from build123d import *

# Parameters (mm, degrees)
SKETCH_1_W          = 60
SKETCH_1_H          = 60
EXTRUDE_1_DEPTH     = 37
SKETCH_2_W          = 56
SKETCH_2_H          = 56
EXTRUDE_2_DEPTH     = 49
CUT_EXTRUDE_1_DEPTH = 49
SKETCH_4_R          = 2
CUT_EXTRUDE_2_DEPTH = 49
FILLET_1_R          = 2
SKETCH_5_R          = 27
CUT_EXTRUDE_3_DEPTH = 1
SKETCH_6_R          = 12
EXTRUDE_3_DEPTH     = 4
SKETCH_7_R          = 4
EXTRUDE_4_DEPTH     = 27
SKETCH_8_W          = 5.291502622
SKETCH_8_H          = 3.956308335
CUT_EXTRUDE_4_DEPTH = 27
FILLET_2_R          = 1
FILLET_3_R          = 3


with BuildPart() as part:
    # Эскиз1 → Бобышка-Вытянуть1 (new body)
    with BuildSketch(Plane.XY):
        with Locations((0.572032188, -6.927630122)):
            Rectangle(SKETCH_1_W, SKETCH_1_H)
    extrude(amount=EXTRUDE_1_DEPTH)

    # Эскиз2 → Бобышка-Вытянуть2 (add)
    with BuildSketch(Plane.XY.offset(37)):
        with Locations((0.572032188, -6.927630122)):
            Rectangle(SKETCH_2_W, SKETCH_2_H)
    extrude(amount=EXTRUDE_2_DEPTH)

    # Эскиз3 → Вырез-Вытянуть1 (cut)
    with BuildSketch(Plane.XY.offset(86)):
        with BuildLine():
            Line((-19.176705154, 17.82110722), (-19.176705154, 21.072369878))
            Line((-19.176705154, 21.072369878), (-27.427967812, 21.072369878))
            Line((-27.427967812, 21.072369878), (-27.427967812, 12.82110722))
            Line((-27.427967812, 12.82110722), (-24.176705154, 12.82110722))
            ThreePointArc((-24.176705154, 12.82110722), (-20.641171248, 14.285573314), (-19.176705154, 17.82110722))
        make_face()
        with BuildLine():
            Line((20.32076953, 17.82110722), (20.32076953, 21.072369878))
            Line((20.32076953, 21.072369878), (28.572032188, 21.072369878))
            Line((28.572032188, 21.072369878), (28.572032188, 12.82110722))
            Line((28.572032188, 12.82110722), (25.32076953, 12.82110722))
            ThreePointArc((25.32076953, 12.82110722), (21.785235624, 14.285573314), (20.32076953, 17.82110722))
        make_face()
        with BuildLine():
            Line((-24.176705154, -26.676367463), (-27.427967812, -26.676367463))
            Line((-27.427967812, -26.676367463), (-27.427967812, -34.927630122))
            Line((-27.427967812, -34.927630122), (-19.176705154, -34.927630122))
            Line((-19.176705154, -34.927630122), (-19.176705154, -31.676367463))
            ThreePointArc((-19.176705154, -31.676367463), (-20.641171248, -28.140833557), (-24.176705154, -26.676367463))
        make_face()
        with BuildLine():
            Line((25.32076953, -26.676367463), (28.572032188, -26.676367463))
            Line((28.572032188, -26.676367463), (28.572032188, -34.927630122))
            Line((28.572032188, -34.927630122), (20.32076953, -34.927630122))
            Line((20.32076953, -34.927630122), (20.32076953, -31.676367463))
            ThreePointArc((20.32076953, -31.676367463), (21.785235624, -28.140833557), (25.32076953, -26.676367463))
        make_face()
    extrude(amount=-CUT_EXTRUDE_1_DEPTH, mode=Mode.SUBTRACT)

    # Эскиз4 → Вырез-Вытянуть2 (cut)
    with BuildSketch(Plane.XY.offset(37)):
        with Locations((-24.176705154, 17.82110722)):
            Circle(SKETCH_4_R)
        with Locations((25.32076953, 17.82110722)):
            Circle(SKETCH_4_R)
        with Locations((-24.176705154, -31.676367463)):
            Circle(SKETCH_4_R)
        with Locations((25.32076953, -31.676367463)):
            Circle(SKETCH_4_R)
    extrude(amount=-CUT_EXTRUDE_2_DEPTH, mode=Mode.SUBTRACT)

    # Скругление1
    fillet_1_edges = [part.edges().sort_by_distance(p)[0] for p in [
        (-19.176705154, 21.072369878, 61.5),
        (-27.427967812, 12.82110722, 61.5),
        (28.572032188, 12.82110722, 61.5),
        (20.32076953, 21.072369878, 61.5),
        (-19.176705154, -34.927630122, 61.5),
        (-27.427967812, -26.676367463, 61.5),
        (28.572032188, -26.676367463, 61.5),
        (20.32076953, -34.927630122, 61.5),
    ]]
    fillet(fillet_1_edges, radius=FILLET_1_R)

    # Эскиз5 → Вырез-Вытянуть3 (cut)
    with BuildSketch(Plane(origin=(0, 0, 0), x_dir=(-1, 0, 0), z_dir=(0, 0, -1))):
        with Locations((-0.572032188, -6.927630122)):
            Circle(SKETCH_5_R)
    extrude(amount=-CUT_EXTRUDE_3_DEPTH, mode=Mode.SUBTRACT)

    # Эскиз6 → Бобышка-Вытянуть3 (add)
    with BuildSketch(Plane(origin=(0, 0, 1), x_dir=(-1, 0, 0), z_dir=(0, 0, -1))):
        with Locations((-0.572032188, 3.072369878)):
            Circle(SKETCH_6_R)
    extrude(amount=EXTRUDE_3_DEPTH)

    # Эскиз7 → Бобышка-Вытянуть4 (add)
    with BuildSketch(Plane(origin=(0, 0, -3), x_dir=(-1, 0, 0), z_dir=(0, 0, -1))):
        with Locations((-0.572032188, 3.072369878)):
            Circle(SKETCH_7_R)
    extrude(amount=EXTRUDE_4_DEPTH)

    # Эскиз8 → Вырез-Вытянуть4 (cut)
    with BuildSketch(Plane(origin=(0, 0, -30), x_dir=(-1, 0, 0), z_dir=(0, 0, -1))):
        with Locations((-0.572032188, 8.050524046)):
            Rectangle(SKETCH_8_W, SKETCH_8_H)
    extrude(amount=-CUT_EXTRUDE_4_DEPTH, mode=Mode.SUBTRACT)

    # Скругление2
    fillet_2_edges = [part.edges().sort_by_distance(p)[0] for p in [
        (28.572032188, -6.927630122, 86),
        (25.946400859, -26.676367463, 86),
        (20.32076953, 18.446738549, 86),
        (0.572032188, 21.072369878, 86),
        (-24.802336483, 12.82110722, 86),
        (-27.427967812, -6.927630122, 86),
        (-19.176705154, -32.301998793, 86),
        (0.572032188, -34.927630122, 86),
        (-26.842181374, 12.235320782, 86),
        (-18.590918716, 20.486583441, 86),
        (-26.842181374, -26.090581026, 86),
        (-18.590918716, -34.341843684, 86),
        (19.734983092, -34.341843684, 86),
        (27.98624575, -26.090581026, 86),
        (19.734983092, 20.486583441, 86),
        (27.98624575, 12.235320782, 86),
        (-20.641171248, 14.285573314, 86),
        (-19.176705154, 18.446738549, 86),
        (21.785235624, 14.285573314, 86),
        (25.946400859, 12.82110722, 86),
        (-20.641171248, -28.140833557, 86),
        (-24.802336483, -26.676367463, 86),
        (21.785235624, -28.140833557, 86),
        (20.32076953, -32.301998793, 86),
    ]]
    fillet(fillet_2_edges, radius=FILLET_2_R)

    # Скругление3
    fillet_3_edges = [part.edges().sort_by_distance(p)[0] for p in [
        (-29.427967812, 23.072369878, 18.5),
        (30.572032188, 23.072369878, 18.5),
        (30.572032188, -36.927630122, 18.5),
        (-29.427967812, -36.927630122, 18.5),
    ]]
    fillet(fillet_3_edges, radius=FILLET_3_R)


solid = part.part
Model file for the job. Use its own axes, mm. A direction names the side the tool comes from. Coordinates: 2 decimals unless noted, no trailing zeros. Order: outer loops, then holes, each group sorted by start corner. A loop starts at its lowest first (then second) coordinate and runs counter-clockwise, first axis right, second up. Notation, with made-up numbers: M 43.25,6 L 65.25,6 A20 cw 65.25,22 Z; hole C 54.5,36 d4. An arc over 180 degrees is marked long. Return JSON: item names as keys, results as strings.
1. Saw through at D-D (x = 9). Give the cut face in (y, z), and give its area (3 significant figures).
Ans:
{"outline": "M -36.93,0 L -32.58,0 L -32.58,1 L -5.47,1 L -5.47,-3 L 11.61,-3 L 11.61,1 L 18.72,1 L 18.72,0 L 23.07,0 L 23.07,37 L 21.07,37 L 21.07,85 A1 ccw 20.07,86 L -33.93,86 A1 ccw -34.93,85 L -34.93,37 L -36.93,37 Z", "area": "4,980 mm^2"}
2. Pull direction X, two halves, no side cores. Call faces 1 (the face through (-25.651, -30.325, 18.759)), 2 (the face through (-20.6, -28.18, 61.34)), 3 (the face through (29.67, -36.07, 18.76)): +X half, -X half, draft (parallel to the pull), parting line (faces both ways), or undercut.
Ans:
{"face 1": "undercut", "face 2": "-X half", "face 3": "+X half"}
3. Saw through at A-A (z = 4.5). Give the cut face in (x, y).
Ans:
{"outline": "M -29.43,-33.93 A3 ccw -26.43,-36.93 L 27.57,-36.93 A3 ccw 30.57,-33.93 L 30.57,20.07 A3 ccw 27.57,23.07 L -26.43,23.07 A3 ccw -29.43,20.07 Z; hole C -24.18,-31.68 d4; hole C -24.18,17.82 d4; hole C 25.32,-31.68 d4; hole C 25.32,17.82 d4"}
4. Saw through at B-B (z = 61.5). Give the cut face in (x, y).
Ans:
{"outline": "M -27.43,-24.68 A2 ccw -25.43,-26.68 L -24.18,-26.68 A5 cw -19.18,-31.68 L -19.18,-32.93 A2 ccw -17.18,-34.93 L 18.32,-34.93 A2 ccw 20.32,-32.93 L 20.32,-31.68 A5 cw 25.32,-26.68 L 26.57,-26.68 A2 ccw 28.57,-24.68 L 28.57,10.82 A2 ccw 26.57,12.82 L 25.32,12.82 A5 cw 20.32,17.82 L 20.32,19.07 A2 ccw 18.32,21.07 L -17.18,21.07 A2 ccw -19.18,19.07 L -19.18,17.82 A5 cw -24.18,12.82 L -25.43,12.82 A2 ccw -27.43,10.82 Z"}
5. Tool access for faces 4 (the face through (-27.428, -7, 61)), 5 (the face through (0, 21.072, 61)), 6 (the face through (21.82, 14.25, 61.34)), 7 (the face through (0.707, -0.925, -16.311)): list every direction of +Z, -Z, +X, -X, +Y, -Y with a clear straight run to the whole face (end or side of a thin tool).
Ans:
{"face 4": "+Z, -X, +Y, -Y", "face 5": "+Z, +X, -X, +Y", "face 6": "+Z, +X, +Y", "face 7": "-Z"}
6. Saw through at C-C (y = -15). Give the cut face in (x, z), and give its area (3 significant figures).
Ans:
{"outline": "M -29.43,0 L -25.19,0 L -25.19,1 L 26.34,1 L 26.34,0 L 30.57,0 L 30.57,37 L 28.57,37 L 28.57,85 A1 ccw 27.57,86 L -26.43,86 A1 ccw -27.43,85 L -27.43,37 L -29.43,37 Z", "area": "4,910 mm^2"}
7. Flat gauge pins, fed straight in: pin 1 (1.4 mm diameter, centred on x = -25, z = 49, fed in from -Y); pin 2 (12 mm diameter, centred on y = 10.5, z = 71, fed in from +X); pin 3 (8 mm diameter, centred on x = -11.5, z = 37.5, fed in from +Y); pin 4 (6 mm diameter, centred on x = -10, z = 54, fed in from +Y). Where does each tip first touch, or does it go through?
Ans:
{"pin 1": "y = -26.68", "pin 2": "x = 28.57", "pin 3": "y = 23.07", "pin 4": "y = 21.07"}
8. Drill centre lines: probe 1 along Y at (x, z) = (-24, 27.5); probe 2 along Y at (x, z) = (-9.5, 46); probe 3 along Z at (x, y) = (21, -10.5). Where is each one in solid material? Low to high.
Ans:
{"probe 1": "-36.93 to -33.67, -29.68 to 15.83, 19.81 to 23.07", "probe 2": "-34.93 to 21.07", "probe 3": "1 to 86"}
